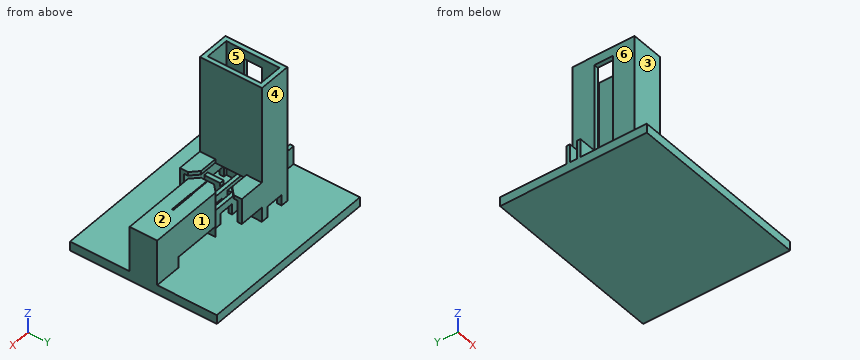
from build123d import *

# Parameters (mm, degrees)
F0_W          = 11.303
F0_H          = 21.463
F0_W_2        = 8.255
F0_H_2        = 18.415
F1_DEPTH      = 50.8
F2_W          = 18.415
F2_H          = 6.35
F3_DEPTH      = 12.7
F4_W          = 6.35
F4_H          = 31.75
F5_DEPTH      = 25.4
F6_W          = 63.5
F6_H          = 50.8
F7_DEPTH      = 3.175
F8_W          = 28.448
F8_H          = 9.525
F9_DEPTH      = 15.875
F11_DEPTH     = 15.875
F12_W         = 35.052
F12_H         = 1.27
F13_DEPTH     = 6.35
F14_W         = 1.27
F14_H         = 1.27
F14_W_2       = 2.3495
F15_DEPTH     = 24.7025
F16_W         = 6.223
F16_H         = 3.81
F16_W_2       = 5.2705
F16_W_3       = 16.383
F17_DEPTH     = 36.1325
F19_DEPTH     = 8.89
F20_T1_DEPTH  = 14.3341495789
F20_T6_DEPTH  = 22.4070747894
F20_T11_DEPTH = 28.9391495789
F20_T16_DEPTH = 22.4070747894
F20_T21_DEPTH = 28.9391495789


# Not quite as in the source:
# - a fillet or chamfer that OpenCascade refuses, or shapes differently, is made with other operations: its cross-section is extruded or revolved along the edge and cut away or added


with BuildPart() as f1:
    # F0 (on Top) → F1 (new body)
    with BuildSketch(Plane.XY):
        Rectangle(F0_W, F0_H)
        Rectangle(F0_W_2, F0_H_2, mode=Mode.SUBTRACT)
    extrude(amount=F1_DEPTH)

    # F2 (on Right) → F3 (cut, symmetric)
    with BuildSketch(Plane.YZ):
        with Locations((0, 12.7)):
            Rectangle(F2_W, F2_H)
    extrude(amount=F3_DEPTH, both=True, mode=Mode.SUBTRACT)

    # F4 (on Right) → F5 (cut)
    with BuildSketch(Plane.YZ):
        with Locations((0, 31.75)):
            Rectangle(F4_W, F4_H)
    extrude(amount=-F5_DEPTH, mode=Mode.SUBTRACT)

    # F6 (on Top) → F7 (join)
    with BuildSketch(Plane.XY):
        with Locations((12.7, 0)):
            Rectangle(F6_W, F6_H)
    extrude(amount=F7_DEPTH)

    # F8 (on face) → F9 (join)
    with BuildSketch(Plane.XY.offset(3.175)):
        with Locations((30.226, 0)):
            Rectangle(F8_W, F8_H)
    extrude(amount=F9_DEPTH)

    # F10 (on face) → F11 (cut, through all)
    with BuildSketch(Plane.XY.offset(19.05)):
        Polygon((11.684, 0.127), (11.684, -0.127), (23.1648, -0.127), (23.1648, -0.254), (31.496, -0.254), (31.496, 0.254), (23.1648, 0.254), (23.1648, 0.127), align=None)
    extrude(amount=-F11_DEPTH, mode=Mode.SUBTRACT)

    # F12 (on face) → F13 (join)
    with BuildSketch(Plane.XY.offset(3.175)):
        with Locations((-1.524, 1.80975)):
            Rectangle(F12_W, F12_H)
        with Locations((-1.524, -1.80975)):
            Rectangle(F12_W, F12_H)
    extrude(amount=F13_DEPTH)

    # F14 (on face) → F15 (cut, through all)
    with BuildSketch(Plane.YZ.offset(5.6515)):
        with Locations((-3.07975, 8.89)):
            Rectangle(F14_W, F14_H)
        with Locations((0, 8.89)):
            Rectangle(F14_W_2, F14_H)
        with Locations((3.07975, 8.89)):
            Rectangle(F14_W, F14_H)
    extrude(amount=-F15_DEPTH, mode=Mode.SUBTRACT)

    # F16 (on face) → F17 (cut, through all)
    with BuildSketch(Plane.XZ.offset(10.7315)):
        with Locations((0, 5.08)):
            Rectangle(F16_W, F16_H)
        with Locations((10.82675, 5.08)):
            Rectangle(F16_W_2, F16_H)
        with Locations((26.7335, 5.08)):
            Rectangle(F16_W_3, F16_H)
    extrude(amount=-F17_DEPTH, mode=Mode.SUBTRACT)

    # F18 (on face) → F19 (join)
    with BuildSketch(Plane.YZ.offset(5.6515)):
        Polygon((-9.2075, 15.875), (-5.3975, 15.875), (-5.3975, 17.145), (-10.7315, 17.145), (-10.7315, 8.255), (-9.2075, 8.255), align=None)
        Polygon((10.7315, 17.145), (5.3975, 17.145), (5.3975, 15.875), (9.2075, 15.875), (9.2075, 8.255), (10.7315, 8.255), align=None)
    extrude(amount=F19_DEPTH)

    # F20: chamfer of 2.54 on 4 edges, made by hand

    # F20_s2 → F20_t1 (cut)
    with BuildSketch(Plane.XY.offset(9.3429252106)):
        Polygon((14.5415, 7.9375), (12.0015, 5.3975), (14.5415, 5.3975), align=None)
        Polygon((12.0015, -5.3975), (14.5415, -7.9375), (14.5415, -5.3975), align=None)
    extrude(amount=F20_T1_DEPTH, mode=Mode.SUBTRACT)


with BuildPart() as f20_tool4:
    # F20_s5 → F20_t6 (new body)
    with BuildSketch(Plane.XY.offset(3.175)):
        Polygon((16.002, -2.2225), (18.542, -4.7625), (16.002, -4.7625), align=None)
    extrude(amount=F20_T6_DEPTH)

    split(bisect_by=Plane.XZ.offset(2.44475), keep=Keep.TOP)


with BuildPart() as f1_1:
    add(f1.part)

    # F20_t3: cut F20_tool4
    add(f20_tool4.part, mode=Mode.SUBTRACT)


with BuildPart() as f20_tool9:
    # F20_s10 → F20_t11 (new body)
    with BuildSketch(Plane.XY.offset(-3.3570747894)):
        Polygon((16.002, -2.2225), (18.542, -4.7625), (16.002, -4.7625), align=None)
    extrude(amount=F20_T11_DEPTH)

    split(bisect_by=Plane.XY.offset(9.525), keep=Keep.TOP)


with BuildPart() as f1_2:
    add(f1_1.part)

    # F20_t8: cut F20_tool9
    add(f20_tool9.part, mode=Mode.SUBTRACT)


with BuildPart() as f20_tool14:
    # F20_s15 → F20_t16 (new body)
    with BuildSketch(Plane.XY.offset(3.175)):
        Polygon((16.002, 2.2225), (18.542, 4.7625), (16.002, 4.7625), align=None)
    extrude(amount=F20_T16_DEPTH)

    split(bisect_by=Plane.XZ.offset(-2.44475), keep=Keep.BOTTOM)


with BuildPart() as f1_3:
    add(f1_2.part)

    # F20_t13: cut F20_tool14
    add(f20_tool14.part, mode=Mode.SUBTRACT)


with BuildPart() as f20_tool19:
    # F20_s20 → F20_t21 (new body)
    with BuildSketch(Plane.XY.offset(-3.3570747894)):
        Polygon((16.002, 2.2225), (18.542, 4.7625), (16.002, 4.7625), align=None)
    extrude(amount=F20_T21_DEPTH)

    split(bisect_by=Plane.XY.offset(9.525), keep=Keep.TOP)


with BuildPart() as f1_4:
    add(f1_3.part)

    # F20_t18: cut F20_tool19
    add(f20_tool19.part, mode=Mode.SUBTRACT)


solid = f1_4.part
Input: part model. Units: mm. Frame: model coordinates. Face numbers are marked on the shaded views. A direction names the side the tool comes from. Coordinates: 2 decimals unless noted, no trailing zeros. Write each loop counter-clockwise with the first axis right and the second up, starting at its lowest first coordinate (ties: lowest second). Pieces come first, ordered by that corner, then holes. Notation, with made-up numbers: M 31,20.25 L 74,20.25 A14 ccw 74,40.25 Z; hole C -15,23.25 d9. An arc over 180 degrees is marked long. Answer as a JSON object with one key per item and string values. Group by question number.
(1) Section B-B on x = -0.5. Output: boundary loops of the cut face in (y, z) (1 decimal), plus the area to 3 significant figures.
(2) Mould query, pull axis X, two halves, no side actions, for the marked faces 4, 5 and 6. Classes: pulls with the +X half, pulls with the -X half, needs draft (parallel to the pull), parting line crosses it, or undercut.
(3) Section C-C on z = 14.5. Output: boundary loops of the cut face in (x, y).
(4) Contact query for flat-ended pins moving along their axis: P1, Ø17, axis at y = -3.5, z = 27.5, coming from the -X side; P2, Ø2, axis at x = 18, z = 7.5, coming from the -Y side; P3, Ø6, axis at x = 10, y = 8.5, coming from the +Z side (3 decimals). Output: stop coordinate, or through.
(5) Section A-A on x = 20. Give the number of separate pieces and of enclosed holes in the cut face, plus the area to 3 significant figures.
(6) Ray query, line 1 along Y through (x, z) = (23.5, 10); line 2 along Y through (x, z) = (-0.5, 14); line 3 along X through (y, z) = (7, 40). Return the intervals inside material, ascending. Write a range as [from, to].
(7) Set-up query: the marked faces 1, 2 and 3. Return all of +Z, -Z, +X, -X, +Y, -Y with unobstructed straight access to the full face (end or side cutting, diameter ignored); none if empty.
Result set:
{
 "1": {"outline": "M -25.4,0 L 25.4,0 L 25.4,3.2 L -25.4,3.2 Z; M -10.7,7 L -9.2,7 L -9.2,50.8 L -10.7,50.8 Z; M -2.4,7 L -1.2,7 L -1.2,9.5 L -2.4,9.5 Z; M 1.2,7 L 2.4,7 L 2.4,9.5 L 1.2,9.5 Z; M 9.2,7 L 10.7,7 L 10.7,50.8 L 9.2,50.8 Z", "area": "301 mm2"},
 "2": {"face 4": "needs draft", "face 5": "undercut", "face 6": "pulls with the -X half"},
 "3": {"outline": "M -5.65,-10.73 L 14.54,-10.73 L 14.54,-9.21 L -5.65,-9.21 Z; M -5.65,9.21 L 14.54,9.21 L 14.54,10.73 L -5.65,10.73 Z; M 16,-2.22 L 18.54,-4.76 L 44.45,-4.76 L 44.45,4.76 L 18.54,4.76 L 16,2.22 L 16,0.13 L 23.16,0.13 L 23.16,0.25 L 31.5,0.25 L 31.5,-0.25 L 23.16,-0.25 L 23.16,-0.13 L 16,-0.13 Z"},
 "4": {"P1": "stops at x = -5.65", "P2": "stops at y = -4.76", "P3": "stops at z = 17.145"},
 "5": {"separate pieces": "3", "enclosed holes": "0", "area": "273 mm2"},
 "6": {"line 1": "y = [-4.76, -0.25], [0.25, 4.76]", "line 2": "y = [-10.73, -9.21], [9.21, 10.73]", "line 3": "x = [-5.65, -4.13], [4.13, 5.65]"},
 "7": {"face 1": "+Z, +X, +Y", "face 2": "+Z, +X, +Y, -Y", "face 3": "+Z, +X, -X, -Y"}
}
